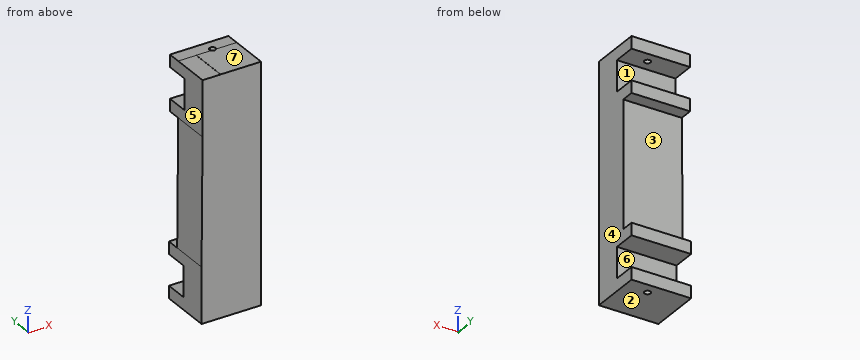
from build123d import *

# Parameters (mm, degrees)
EXTRUDE_1_DEPTH           = 30
SKETCH_2_W                = 20
SKETCH_2_H                = 15
SKETCH_2_W_2              = 70
SKETCH_2_H_2              = 10
EXTRUDE_4_DEPTH           = 70
SKETCH_5_R                = 2.8
CUT_EXTRUDE_3_DEPTH       = 5
SKETCH_6_R                = 2.8
CUT_EXTRUDE_4_DEPTH       = 5
PATTERN_LINEAR_1_COUNT    = 3
PATTERN_LINEAR_1_PITCH    = 19
SKETCH_14_W               = 30
SKETCH_14_H               = 20
EXTRUDE_16_DEPTH          = 8.5
EXTRUDE_17_DEPTH          = 8.5
EXTRUDE_18_DEPTH          = 8.5
SKETCH_15_W               = 140
SKETCH_15_H               = 160
EXTRUDE_21_DEPTH          = 10
SKETCH_17_W               = 140
SKETCH_17_H               = 160
EXTRUDE_22_DEPTH          = 15
CUT_EXTRUDE_8_REACH       = 328.336
SKETCH_20_R               = 2
CUT_EXTRUDE_10_REACH      = 267.273
CUT_EXTRUDE_11_REACH      = 267.358
SKETCH_22_R               = 2
SKETCH_23_R               = 2.8
CUT_EXTRUDE_12_DEPTH      = 5
SKETCH_24_R               = 1.9
CUT_EXTRUDE_13_DEPTH      = 5
CUT_EXTRUDE_16_DEPTH      = 251.685617404
CUT_EXTRUDE_16_DEPTH_BACK = 251.685617404
CUT_EXTRUDE_17_DEPTH      = 15


with BuildPart() as part:
    # 草图1 → 凸台-拉伸1 (new body)
    with BuildSketch(Plane(origin=(0, 0, 0), x_dir=(0, 0, -1), z_dir=(1, 0, 0))):
        Polygon((-20.255776875, 11.348042253), (-20.255776875, -3.651957747), (-0.255776875, -3.651957747), (-0.255776875, 11.348042253), (97.744223125, 11.348042253), (97.744223125, -3.651957747), (117.744223125, -3.651957747), (117.744223125, 11.348042253), (125.744223125, 11.348042253), (125.744223125, -13.651957747), (-28.255776875, -13.651957747), (-28.255776875, 11.348042253), align=None)
    extrude(amount=EXTRUDE_1_DEPTH)

    # 草图2 → 凸台-拉伸4 (add)
    with BuildSketch(Plane.ZY):
        Polygon((-125.744223125, 11.348042253), (-117.744223125, 11.348042253), (-117.744223125, 16.348042253), (-132.744223125, 16.348042253), (-132.744223125, -13.651957747), (-125.744223125, -13.651957747), align=None)
        Polygon((-117.744223125, -13.651957747), (-117.744223125, -3.651957747), (-117.744223125, 11.348042253), (-125.744223125, 11.348042253), (-125.744223125, -13.651957747), align=None)
        Polygon((-97.744223125, -3.651957747), (-117.744223125, -3.651957747), (-117.744223125, -13.651957747), (28.255776875, -13.651957747), (28.255776875, 11.348042253), (20.255776875, 11.348042253), (20.255776875, -3.651957747), (0.255776875, -3.651957747), (0.255776875, 11.348042253), (-97.744223125, 11.348042253), align=None)
        with Locations((-107.744223125, 3.848042253)):
            Rectangle(SKETCH_2_W, SKETCH_2_H)
        with Locations((10.255776875, 3.848042253)):
            Rectangle(SKETCH_2_W, SKETCH_2_H)
        Polygon((28.255776875, 11.348042253), (28.255776875, -13.651957747), (53.255776875, -13.651957747), (53.255776875, -3.651957747), (53.255776875, 11.348042253), align=None)
        with Locations((88.255776875, -8.651957747)):
            Rectangle(SKETCH_2_W_2, SKETCH_2_H_2)
    extrude(amount=EXTRUDE_4_DEPTH)

    # 草图5 → 切除-拉伸3 (cut)
    with BuildSketch(Plane(origin=(0, 16.348042253, 0), x_dir=(1, 0, 0), z_dir=(0, 1, 0))):
        with Locations(Location((-51, 125.244223125, 0), (0, 0, 270))):
            Circle(SKETCH_5_R)
        with Locations(Location((-19, 125.244223125, 0), (0, 0, 270))):
            Circle(SKETCH_5_R)
    extrude(amount=-CUT_EXTRUDE_3_DEPTH, mode=Mode.SUBTRACT)

    # 草图6 → 切除-拉伸4 (cut)
    with BuildSketch(Plane(origin=(0, -3.651957747, 0), x_dir=(1, 0, 0), z_dir=(0, 1, 0))):
        with Locations(Location((-55, -112.316244648, 0), (0, 0, 270))):
            Circle(SKETCH_6_R)
        with Locations(Location((-15, -112.316244648, 0), (0, 0, 270))):
            Circle(SKETCH_6_R)
    cut_extrude_4 = extrude(amount=-CUT_EXTRUDE_4_DEPTH, mode=Mode.SUBTRACT)

    # 阵列(线性)1: 切除-拉伸4 ×3
    with Locations(*[(0, 0, -i * PATTERN_LINEAR_1_PITCH) for i in range(1, PATTERN_LINEAR_1_COUNT)]):
        add(cut_extrude_4, mode=Mode.SUBTRACT)

    # 草图14 → 凸台-拉伸16 (add)
    with BuildSketch(Plane(origin=(0, -3.651957747, 0), x_dir=(1, 0, 0), z_dir=(0, 1, 0))):
        with Locations((15, -10.255776875)):
            Rectangle(SKETCH_14_W, SKETCH_14_H)
        with Locations((15, 107.744223125)):
            Rectangle(SKETCH_14_W, SKETCH_14_H)
    extrude(amount=EXTRUDE_16_DEPTH)

    # 草图9 → 凸台-拉伸17 (add)
    with BuildSketch(Plane(origin=(0, 11.348042253, 0), x_dir=(1, 0, 0), z_dir=(0, 1, 0))):
        Polygon((-8.658071854, 117.744223125), (-8.658071854, 125.744223125), (0, 125.744223125), (30, 125.744223125), (30, 117.744223125), (0, 117.744223125), (0, 97.744223125), (30, 97.744223125), (30, 89.744223125), (-8.658071854, 89.744223125), align=None)
    extrude(amount=EXTRUDE_17_DEPTH)

    # 草图13 → 凸台-拉伸18 (add)
    with BuildSketch(Plane(origin=(0, 11.348042253, 0), x_dir=(1, 0, 0), z_dir=(0, 1, 0))):
        Polygon((30, -0.255776875), (30, 7.744223125), (-8, 7.744223125), (-8, -28.176051311), (30, -28.255776875), (30, -20.255776875), (0, -20.255776875), (0, -0.255776875), align=None)
    extrude(amount=EXTRUDE_18_DEPTH)

    # 草图15 → 凸台-拉伸21 (add)
    with BuildSketch(Plane(origin=(0, -3.651957747, 0), x_dir=(1, 0, 0), z_dir=(0, 1, 0))):
        with Locations((-140, -43.255776875)):
            Rectangle(SKETCH_15_W, SKETCH_15_H)
    extrude(amount=-EXTRUDE_21_DEPTH)

    # 草图17 → 凸台-拉伸22 (add)
    with BuildSketch(Plane(origin=(0, -3.651957747, 0), x_dir=(1, 0, 0), z_dir=(0, 1, 0))):
        with Locations((-140, -43.255776875)):
            Rectangle(SKETCH_17_W, SKETCH_17_H)
    extrude(amount=EXTRUDE_22_DEPTH)

    # 草图20 → 切除-拉伸8 (cut, up to next)
    with BuildSketch(Plane(origin=(0, 0, -125.744223125), x_dir=(-1, 0, 0), z_dir=(0, 0, -1)), mode=Mode.PRIVATE) as cut_extrude_8_sk1:
        with Locations(Location((-15, 12.498042253, 0), (0, 0, 90))):
            Circle(SKETCH_20_R)
    cut_extrude_8_tool1 = extrude(cut_extrude_8_sk1.sketch, amount=-CUT_EXTRUDE_8_REACH, mode=Mode.PRIVATE) & part.part
    add(cut_extrude_8_tool1.solids().sort_by_distance((15, 12.498042, -125.744223))[0], mode=Mode.SUBTRACT)

    # 切除-拉伸10: up to this plane
    cut_extrude_10_end = Plane(origin=(30, 11.348042253, 20.255776875), z_dir=(0, 0, 1))
    # 草图21 → 切除-拉伸10 (cut, up to the surface)
    with BuildSketch(Plane(origin=(-0.059149469, 0, 28.192711542), x_dir=(0.9999977991189155, 0, 0.0020980365404790436), z_dir=(-0.0020980365404790436, 0, 0.9999977991189156)), mode=Mode.PRIVATE) as cut_extrude_10_sk1:
        with BuildLine():
            ThreePointArc((17.059215626, 12.498042253), (14.456145827, 14.404952533), (13.422908809, 11.348042253))
            Line((13.422908809, 11.348042253), (16.695522443, 11.348042253))
            ThreePointArc((16.695522443, 11.348042253), (16.966125906, 11.894972454), (17.059215626, 12.498042253))
        make_face()
    cut_extrude_10_tool1 = split(extrude(cut_extrude_10_sk1.sketch, amount=-CUT_EXTRUDE_10_REACH, mode=Mode.PRIVATE), bisect_by=cut_extrude_10_end, keep=Keep.BOTH, mode=Mode.PRIVATE)
    add(cut_extrude_10_tool1.solids().sort_by_distance((15.000033, 12.773192, 28.224306))[0], mode=Mode.SUBTRACT)

    # 草图22 → 切除-拉伸11 (cut, up to next)
    with BuildSketch(Plane.XY.offset(28.255776875), mode=Mode.PRIVATE) as cut_extrude_11_sk1:
        with Locations(Location((15, 12.498042253, 0), (0, 0, 90))):
            Circle(SKETCH_22_R)
    cut_extrude_11_tool1 = extrude(cut_extrude_11_sk1.sketch, amount=-CUT_EXTRUDE_11_REACH, mode=Mode.PRIVATE) & part.part
    add(cut_extrude_11_tool1.solids().sort_by_distance((15, 12.498042, 28.255777))[0], mode=Mode.SUBTRACT)

    # 草图23 → 切除-拉伸12 (cut)
    with BuildSketch(Plane(origin=(0, 11.348042253, 0), x_dir=(1, 0, 0), z_dir=(0, 1, 0))):
        with Locations(Location((-194, -93.255776875, 0), (0, 0, 270))):
            Circle(SKETCH_23_R)
        with Locations(Location((-86, -93.255776875, 0), (0, 0, 270))):
            Circle(SKETCH_23_R)
    extrude(amount=-CUT_EXTRUDE_12_DEPTH, mode=Mode.SUBTRACT)

    # 草图24 → 切除-拉伸13 (cut)
    with BuildSketch(Plane(origin=(0, 11.348042253, 0), x_dir=(1, 0, 0), z_dir=(0, 1, 0))):
        with Locations(Location((-196.5, 26.744223125, 0), (0, 0, 270))):
            Circle(SKETCH_24_R)
        with Locations(Location((-83.5, 26.744223125, 0), (0, 0, 270))):
            Circle(SKETCH_24_R)
        with Locations(Location((-196.5, -47.555776875, 0), (0, 0, 270))):
            Circle(SKETCH_24_R)
        with Locations(Location((-83.5, -47.555776875, 0), (0, 0, 270))):
            Circle(SKETCH_24_R)
    extrude(amount=-CUT_EXTRUDE_13_DEPTH, mode=Mode.SUBTRACT)

    # 草图26 → 切除-拉伸16 (cut, two sides: drawn at the far end of the back side and taken through both)
    with BuildSketch(Plane(origin=(0, 19.848042253, 0), x_dir=(1, 0, 0), z_dir=(0, 1, 0)).offset(-CUT_EXTRUDE_16_DEPTH_BACK)):
        Polygon((-8, 7.744223125), (-8.658071854, 89.744223125), (-8.658071854, 125.744223125), (3.217660612, 125.744223125), (3.802444891, 150.192522069), (-171.612640653, 166.525859149), (-482.190724596, -91.141473661), (-210.719247924, -353.972429265), (3.510052751, -124.506752876), (3.712106974, -28.200623793), (-8, -28.176051311), align=None)
    extrude(amount=CUT_EXTRUDE_16_DEPTH + CUT_EXTRUDE_16_DEPTH_BACK, mode=Mode.SUBTRACT)

    # 草图27 → 切除-拉伸17 (cut)
    with BuildSketch(Plane(origin=(0, 19.848042253, 0), x_dir=(1, 0, 0), z_dir=(0, 1, 0))):
        Polygon((-11.220288102, -0.255776875), (-9.170863609, -20.255776875), (0, -20.255776875), (0, -0.255776875), align=None)
        Polygon((-8.658071854, 97.744223125), (0, 97.744223125), (0, 117.744223125), (-8.658071854, 104.132040921), align=None)
        Polygon((-16.859481318, 117.744223125), (-12.721063711, 97.744223125), (-8.658071854, 104.132040921), (-8.658071854, 117.744223125), align=None)
        Polygon((-8.658071854, 104.132040921), (0, 117.744223125), (-8.658071854, 117.744223125), align=None)
    extrude(amount=-CUT_EXTRUDE_17_DEPTH, mode=Mode.SUBTRACT)


solid = part.part
Geometry: final body of the model. Coordinates: model frame, mm. Face numbers are marked on the shaded views. A direction names the side the tool comes from. Give positions to 0.01 mm unless a question says otherwise; leave off trailing zeros. Write each loop counter-clockwise with the first axis right and the second up, starting at its lowest first coordinate (ties: lowest second). Pieces come first, ordered by that corner, then holes. Notation, with made-up numbers: M -28.75,37.25 L 20.25,37.25 A12 cw 20.25,52.25 Z; hole C 53,-38 d2. An arc over 180 degrees is marked long. Answer in a Markdown table with one row per item. Add a question column.
(1) Section D-D on x = -2. Return loops of the section in (y, z), and give its area (3 significant figures).
(2) Mould query, pull axis Z, two halves, no side actions, for the marked faces 1, 2, 3 and 4. Classes: +Z half, -Z half, draft (parallel to the pull), parting line (faces both ways), or undercut.
(3) Section C-C on z = 12. Return loops of the section in (x, y).
(4) Reachability of the marked faces 5, 6 and 7 from +Z, -Z, +X, -X, +Y, -Y: full face, straight path, thin tool, end or side. Return the list, or none.
(5) Section A-A on y = 8. Return loops of the section in (x, z).
(6) First-contact query: pin 1 (9.5 mm diameter, centred on x = 12, y = 17.5, fed in from +Z); pin 2 (6 mm diameter, centred on x = 5, z = -104, fed in from +Y); pin 3 (3.5 mm diameter, centred on x = 15, y = 12.5, fed in from +Z). Flat tips, straight axial feed; report the tip coordinate or a pass-through.
(7) Ray query, line 1 (Z direction, x = -2.5, y = 18); line 2 (Z direction, x = 1, y = 6); line 3 (Y direction, x = 15, z = 25.75). Return the intervals inside material, ascending.
Result set:
| question | item | result |
|---|---|---|
| 1 | outline | M -13.65,-125.74 L 19.85,-125.74 L 19.85,-117.74 L 4.85,-117.74 L 4.85,-97.74 L 19.85,-97.74 L 19.85,-89.74 L 11.35,-89.74 L 11.35,-7.74 L 19.85,-7.74 L 19.85,0.26 L 4.85,0.26 L 4.85,20.26 L 19.85,20.26 L 19.85,28.19 L -13.65,28.19 Z |
| 1 | area | 3,860 mm^2 |
| 2 | face 1 | undercut |
| 2 | face 2 | -Z half |
| 2 | face 3 | undercut |
| 2 | face 4 | draft |
| 3 | outline | M -8,-13.65 L 30,-13.65 L 30,4.85 L -8,4.85 Z |
| 4 | face 5 | +Z, -X, +Y, -Y |
| 4 | face 6 | +X, -X, +Y |
| 4 | face 7 | +Z, +X, -X, +Y, -Y |
| 5 | outline | M -8.66,-125.74 L 30,-125.74 L 30,-117.74 L -8.66,-117.74 Z; M -8.66,-97.74 L 30,-97.74 L 30,0.26 L -8,0.26 L -8,-7.74 L -8.66,-89.74 Z; M -8,20.26 L 30,20.26 L 30,28.26 L 3.71,28.26 L 3.71,28.2 L -8,28.18 Z |
| 6 | pin 1 | stops at z = 28.23 |
| 6 | pin 2 | stops at y = 4.85 |
| 6 | pin 3 | stops at z = 0.26 |
| 7 | line 1 | z = -125.74 to -117.74, -97.74 to -89.74, -7.74 to 0.26, 20.26 to 28.19 |
| 7 | line 2 | z = -125.74 to -117.74, -97.74 to 0.26, 20.26 to 28.19 |
| 7 | line 3 | y = -13.65 to 10.5, 14.5 to 19.85 |
